Geometry check sheet. Reference: drawing and pictorial views, mm from the part's lowest x, y, z. Give positions to 0.01 mm unless a question says otherwise; leave off trailing zeros. Write each loop counter-clockwise with the first axis right and the second up, starting at its lowest first coordinate (ties: lowest second). Pieces come first, ordered by that corner, then holes. Notation, with made-up numbers: (75, 15) -> (130, 15) arc R26 ccw to (130, 41) -> close; hole circle Ø3 at (61, -1.5). An arc over 180 degrees is marked (long way). Use a Markdown table: item, result. Add a question column.
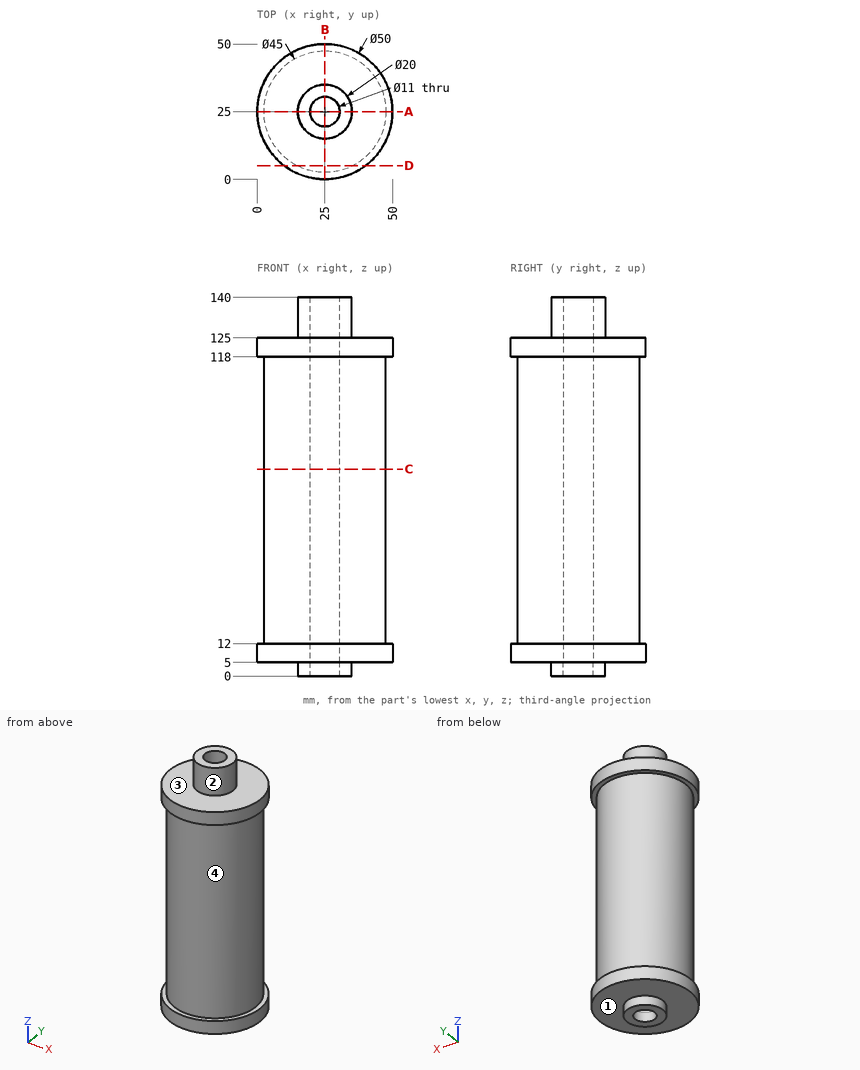
1) Sectioned sample at D-D, the plane y = 5. Enter the section's corners in (x, z), and give its area (3 significant figures).
2) Draft check along Z on the marked faces 1, 2, 3 and 4. Enter one of: +Z half, -Z half, draft (parallel to the pull), parting line (faces both ways), or undercut.
3) Material ranges on probe 1 along Y at (x, z) = (25, 3); probe 2 along X at (y, z) = (25, 98), recorded low to high. Write a range as [from, to].
4) Sectioned sample at A-A, the plane y = 25. Enter the section's corners in (x, z), and give its area (3 significant figures).
5) Gauge pin test, flat ends, axial feed: P1, Ø1.5, axis at x = 32.5, z = 102.5, coming from the -Y side; P2, Ø1.5, axis at x = 29, z = 102.5, coming from the -Y side; P3, Ø9, axis at x = 25, y = 25, coming from the -Z side (1 decimal); P4, Ø3, axis at x = 18, z = 116, coming from the -Y side. Record the tip position at first contact, or that the pin passes through.
6) Sectioned sample at C-C, the plane z = 76.5. Enter the section's corners in (x, y).
Check values:
| question | item | result |
|---|---|---|
| 1 | outline | (10, 5) -> (40, 5) -> (40, 12) -> (35.31, 12) -> (35.31, 118) -> (40, 118) -> (40, 125) -> (10, 125) -> (10, 118) -> (14.69, 118) -> (14.69, 12) -> (10, 12) -> close |
| 1 | area | 2,610 mm² |
| 2 | face 1 | -Z half |
| 2 | face 2 | draft |
| 2 | face 3 | +Z half |
| 2 | face 4 | undercut |
| 3 | probe 1 | [15, 19.5], [30.5, 35] |
| 3 | probe 2 | [2.5, 19.5], [30.5, 47.5] |
| 4 | outline | (0, 5) -> (15, 5) -> (15, 0) -> (19.5, 0) -> (19.5, 140) -> (15, 140) -> (15, 125) -> (0, 125) -> (0, 118) -> (2.5, 118) -> (2.5, 12) -> (0, 12) -> close; (30.5, 0) -> (35, 0) -> (35, 5) -> (50, 5) -> (50, 12) -> (47.5, 12) -> (47.5, 118) -> (50, 118) -> (50, 125) -> (35, 125) -> (35, 140) -> (30.5, 140) -> close |
| 4 | area | 4,330 mm² |
| 5 | P1 | y = 3.54 |
| 5 | P2 | y = 2.74 |
| 5 | P3 | through |
| 5 | P4 | y = 3.18 |
| 6 | outline | circle Ø45 at (25, 25); hole circle Ø11 at (25, 25) |
